Geometry: final body of the model. Coordinates: model frame, mm. A direction names the side the tool comes from. Give positions to 0.01 mm unless a question says otherwise; leave off trailing zeros. Write each loop counter-clockwise with the first axis right and the second up, starting at its lowest first coordinate (ties: lowest second). Pieces come first, ordered by that corner, then holes. Notation, with made-up numbers: M 49.5,76.5 L 93.5,76.5 A25 cw 93.5,107.5 Z; hole C 74,10.5 d4. An arc over 180 degrees is marked long. One line per question, with ' | ' between items.
from build123d import *

# Parameters (mm, degrees)
F0_W     = 101.6
F0_H     = 50.8
F1_DEPTH = 50
F3_DEPTH = 25.4
F4_R     = 6.35
F5_DEPTH = 50.001
F6_R     = 3.175


with BuildPart() as f1:
    # F0 (on Front) → F1 (new body)
    with BuildSketch(Plane.XZ):
        with Locations((50.8, 25.4)):
            Rectangle(F0_W, F0_H)
    extrude(amount=F1_DEPTH)

    # F2 (on face) → F3 (cut)
    with BuildSketch(Plane.XY.offset(50.8)):
        with BuildLine():
            Line((101.6, -50), (101.6, -24.6))
            ThreePointArc((101.6, -24.6), (83.6394877579, -32.0394877579), (76.2, -50))
            Line((76.2, -50), (101.6, -50))
        make_face()
        with BuildLine():
            ThreePointArc((76.2, -50), (101.6, -75.4), (127, -50))
            ThreePointArc((127, -50), (119.5605122421, -32.0394877579), (101.6, -24.6))
            Line((101.6, -24.6), (101.6, -50))
            Line((101.6, -50), (76.2, -50))
        make_face()
    extrude(amount=-F3_DEPTH, mode=Mode.SUBTRACT)

    # F4 (on face) → F5 (cut, through all)
    with BuildSketch(Plane.XZ.offset(50)):
        with Locations((76.2, 38.1)):
            Circle(F4_R)
    extrude(amount=-F5_DEPTH, mode=Mode.SUBTRACT)

    # F6 (on face) → F7 (revolve)
    with BuildSketch(Plane.YZ.offset(101.6)):
        with Locations((-43.65, 6.35)):
            Circle(F6_R)
    revolve(axis=Axis((101.6, -25, 6.2950919382), (0, 0, 1)))


solid = f1.part
(1) Cut plane D-D, the plane z = 15.5. Return loops of the section in (x, y).
Working result:
outline: M 0,-50 L 101.6,-50 L 101.6,0 L 0,0 Z
(2) Cut plane C-C, the plane y = -31.5. Count the separate pieces of the cut face and the enclosed holes in it, then the cut area to 3 significant figures.
Working result:
separate pieces: 2 | enclosed holes: 1 | area: 4,630 mm^2
(3) First-contact query: P1, Ø7.5, axis at x = 95, y = -37, coming from the +Z side; P2, Ø5, axis at y = -24, z = 9, coming from the +X side. Flat tips, straight axial feed; report the tip coordinate or a pass-through.
Working result:
P1: stops at z = 25.4 | P2: stops at x = 123.41
(4) Set-up query: faces 1 (the face through (92, -40, 25.4)), 2 (the face through (39, -50, 26)). Return all of +Z, -Z, +X, -X, +Y, -Y with unobstructed straight access to the full face (end or side cutting, diameter ignored); none if empty.
Working result:
face 1: +Z, +X, -Y | face 2: +Z, -Z, +X, -X, -Y
(5) Cut plane A-A, the plane x = 78.5. Return loops of the section in (y, z), then the cut area to 3 significant figures.
Working result:
outline: M -50,0 L 0,0 L 0,32.18 L -39.44,32.18 L -39.44,25.4 L -50,25.4 Z; M -39.44,44.02 L 0,44.02 L 0,50.8 L -39.44,50.8 Z | area: 1,800 mm^2
(6) Material intervals for L1, parallel to Z at x = 76.2, y = -24.5; L2, parallel to X at y = -7, z = 31; L3, parallel to X at y = -38, z = 38, sorted ascending. Write a range as [from, to].
Working result:
L1: z = [0, 31.75], [44.45, 50.8] | L2: x = [0, 101.6] | L3: x = [0, 69.85]
(7) Cut plane B-B, the plane z = 38.1. Return loops of the section in (x, y).
Working result:
outline: M 0,-50 L 69.85,-50 L 69.85,0 L 0,0 Z; M 82.55,-33.2 A25.4 cw 101.6,-24.6 L 101.6,0 L 82.55,0 Z
